Autodesk Inventor part; units mm, degrees
ref_plane "YZ Plane" through (0, 0, 0) normal (1, 0, 0) x (0, 1, 0)
ref_plane "XZ Plane" through (0, 0, 0) normal (0, 1, 0) x (-1, 0, 0)
ref_plane "XY Plane" through (0, 0, 0) normal (0, 0, 1) x (1, 0, 0)
sketch "Эскиз1" plane through (0, 0, 0) normal (0, 0, 1) x (1, 0, 0)
  circle A0 centre (0, 0) radius 12.5
  line L0 (0, -12.5) -> (280, -12.5)
  line L1 (280, -12.5) -> (280, 12.5)
  line L2 (280, 12.5) -> (0, 12.5)
  line L3 (0, 12.5) -> (0, -12.5)
  circle A1 centre (280, 0) radius 12.5
  circle A2 centre (0, 0) radius 7
  circle A3 centre (280, 0) radius 7
  circle A4 centre (0, 0) radius 4
  circle A5 centre (280, 0) radius 3
  circle A6 centre (287, 0) radius 1.5
  circle A7 centre (280, 7) radius 1.5
  circle A8 centre (280, -7) radius 1.5
  circle A9 centre (287, 0) radius 1.5
  line L4 (138, 12.5) -> (142, 12.5)
  line L5 (142, 12.5) -> (142, 0)
  line L6 (142, 0) -> (138, 0)
  line L7 (138, 0) -> (138, 12.5)
  point P0 (280, -12.5)
  point P1 (140, 12.5)
  point P2 (140, 12.5)
  point P3 (142, 12.5)
  point P4 (140, 0)
  dimension "d0" = 25
  dimension "d1" = 280
  dimension "d2" = 14
  dimension "d3" = 14
  dimension "d8" = 8
  dimension "d9" = 6
  dimension "d10" = 3
  dimension "d11" = 3
  dimension "d12" = 3
  dimension "d13" = 3
  dimension "d16" = 0
  dimension "d17" = 4
  dimension "d26" = 140
extrude "Выдавливание1" add sketch "Эскиз1" along normal blind 4 contours A0 L3 A2 | A0 L2 L7 L6 L5 A1 L0 | L3 A2 A0 | A2 L3 A4 | L3 A4 A2 | A1 L1 A7 A3 A8 | L1 A8 A3 A6 A7 A1 | A3 A7 L1 A5 A8 | L1 A5 A7 A3 A6 A8
sketch "Эскиз2" plane through (0, 0, 4) normal (0, 0, 1) x (1, 0, 0)
  line L0 (152, 23.4347) -> (359.1429, 23.4347)
  line L1 (359.1429, 23.4347) -> (359.1429, -33.9487)
  line L2 (359.1429, -33.9487) -> (152, -33.9487)
  line L3 (152, -33.9487) -> (152, 23.4347)
  line L4 (142, 12.5) -> (142, 0)
  point P0 (0, 0)
  dimension "d18" = 10
extrude "Выдавливание2" cut sketch "Эскиз2" against normal blind 10
fillet "Сопряжение1" radius 2 2 edges at (152, 12.5, 2) (152, -12.5, 2)
sketch "Эскиз3" plane through (0, 0, 4) normal (0, 0, 1) x (1, 0, 0)
  line L0 (138, 12.5) -> (0, 12.5)
  line L1 (67, 12.5) -> (71, 12.5)
  line L2 (71, 12.5) -> (71, 0)
  line L3 (71, 0) -> (67, 0)
  line L4 (67, 0) -> (67, 12.5)
  point P0 (0, 0)
  point P1 (69, 12.5)
  point P2 (69, 12.5)
  point P3 (71, 12.5)
  dimension "d22" = 0
  dimension "d23" = 4
extrude "Выдавливание3" cut sketch "Эскиз3" against normal blind 10
properties material "Дерево (вишня)"
Could you check a few things on this model? Use its own coordinates, in mm. A direction names the side the tool comes from. Coordinates: 2 decimals unless noted, no trailing zeros. Write each loop counter-clockwise with the first axis right and the second up, starting at its lowest first coordinate (ties: lowest second). Pieces come first, ordered by that corner, then holes. Notation, with made-up numbers: (-27.75, 55.5) - (27.25, 55.5) arc R25 ccw to (27.25, 88.5) - close; hole circle Ø10 at (18.25, 61). An arc over 180 degrees is marked (long way). Put each result on its own line as item: value. Start each with the question number.
Q1. Please list where these lines run through material, in increasing order: L1, parallel to Y at x = 0, z = 1.15; L2, parallel to X at y = 1, z = 3; L3, parallel to X at y = 3.5, z = 3.65.
Q2. I want a section at A-A on z = 2. Write out the boundary of the cut face in (x, y), plus the area to 3 significant figures.
Q3. I'm going to push flat-ended pins straight in: P1, Ø1.5, axis at y = 2, z = 0.5, coming from the -X side; P2, Ø2, axis at y = 8.5, z = 2.5, coming from the -X side. Where does each tip first touch, or does it pass through?
Q4. Which directions (+Z, -Z, +X, -X, +Y, -Y) give clear straight access to the entire face, cutting with the end or side of a thin tool? Please do faces 1 (the flat face through (34, 12.5, 2)), 2 (the flat face through (142, 6, 2)).
Q5. Thinking about a two-plate mould opening in Y: for faces 3 (the cylindrical face through (-0.867, 3.905, 1.972)), 4 (the cylindrical face through (-12.497, -0.275, 1.972)), 5 (the flat face through (67, 6, 2)), which applies, pulls with the +Y half, pulls with the -Y half, needs draft (parallel to the pull), parting line crosses it, or undercut?
Checks:
1. L1: -12.5 to -4, 4 to 12.5
1. L2: -12.46 to -3.87, 3.87 to 67, 71 to 138, 142 to 152
1. L3: -12 to -1.94, 1.94 to 67, 71 to 138, 142 to 152
2. outline: (0, -12.5) - (150, -12.5) arc R2 ccw to (152, -10.5) - (152, 10.5) arc R2 ccw to (150, 12.5) - (142, 12.5) - (142, 0) - (138, 0) - (138, 12.5) - (71, 12.5) - (71, 0) - (67, 0) - (67, 12.5) - (0, 12.5) arc R12.5 ccw to start; hole circle Ø8 at (0, 0)
2. area: 3,890 mm²
3. P1: x = -12.44
3. P2: x = -10
4. face 1: +Z, -Z, +X, -X, +Y
4. face 2: +Z, -Z, +Y
5. face 3: undercut
5. face 4: parting line crosses it
5. face 5: needs draft
